Part model, mm, in its own coordinate system. A direction names the side the tool comes from. Round coordinates to 2 decimals unless told otherwise and drop trailing zeros. Write each loop counter-clockwise with the first axis right and the second up, starting at its lowest first coordinate (ties: lowest second). Pieces come first, ordered by that corner, then holes.
```python
from build123d import *

# Parameters (mm, degrees)
F0_R     = 6
F1_DEPTH = 10


with BuildPart() as f1:
    # F0 (on Front) → F1 (new body)
    with BuildSketch(Plane.XZ):
        with BuildLine():
            Line((0, 15), (0, 0))
            Line((0, 0), (55, 0))
            Line((55, 0), (80, 0))
            Line((80, 0), (80, 40))
            Line((80, 40), (70, 40))
            Line((70, 40), (70, 74.051529))
            ThreePointArc((70, 74.051529), (66.311166, 78.381983), (60.857511, 80))
            Line((60.857511, 80), (10, 80))
            Line((10, 80), (10, 15))
            Line((10, 15), (0, 15))
        make_face()
        with Locations((30, 15.13609)):
            Circle(F0_R, mode=Mode.SUBTRACT)
        with Locations((55, 15)):
            Circle(F0_R, mode=Mode.SUBTRACT)
        with Locations((30, 40)):
            Circle(F0_R, mode=Mode.SUBTRACT)
        with Locations((30, 65.102487)):
            Circle(F0_R, mode=Mode.SUBTRACT)
        with Locations((55, 40)):
            Circle(F0_R, mode=Mode.SUBTRACT)
        with Locations((55, 65.307461)):
            Circle(F0_R, mode=Mode.SUBTRACT)
    extrude(amount=F1_DEPTH)


solid = f1.part
```
Q1. Drop a flat-ended pin along its axis: pin 1 (5 mm diameter, centred on x = 6.5, y = -5.5, fed in from +Z). Give the stop position or say it passes through.
Values follow:
pin 1: stops at z = 15
Q2. Cut at B-B on z = 11. Write the cut outline in (x, y).
Values follow:
outline: (0, -10) - (25.65, -10) - (25.65, 0) - (0, 0) - close; (34.35, -10) - (50.53, -10) - (50.53, 0) - (34.35, 0) - close; (59.47, -10) - (80, -10) - (80, 0) - (59.47, 0) - close
Q3. Wall check: L1, parallel to Z at x = 55, y = -4.25; L2, parallel to Z at x = 30, y = -5.25; L3, parallel to X at y = -1, z = 41. Give the ranges that are in metal, low to high.
Values follow:
L1: z = 0 to 9, 21 to 34, 46 to 59.31, 71.31 to 80
L2: z = 0 to 9.14, 21.14 to 34, 46 to 59.1, 71.1 to 80
L3: x = 10 to 24.08, 35.92 to 49.08, 60.92 to 70
Q4. Cut at A-A on x = 55. Write the cut outline in (y, z), plus the area to 3 significant figures.
Values follow:
outline: (-10, 0) - (0, 0) - (0, 9) - (-10, 9) - close; (-10, 21) - (0, 21) - (0, 34) - (-10, 34) - close; (-10, 46) - (0, 46) - (0, 59.31) - (-10, 59.31) - close; (-10, 71.31) - (0, 71.31) - (0, 80) - (-10, 80) - close
area: 440 mm2
Q5. Cut at D-D on z = 36.5. Write the cut outline in (x, y), plus the area to 3 significant figures.
Values follow:
outline: (10, -10) - (25.13, -10) - (25.13, 0) - (10, 0) - close; (34.87, -10) - (50.13, -10) - (50.13, 0) - (34.87, 0) - close; (59.87, -10) - (80, -10) - (80, 0) - (59.87, 0) - close
area: 505 mm2
Q6. Cut at C-C on y = -7.25. Write the cut outline in (x, z), plus the area to 3 significant figures.
Values follow:
outline: (0, 0) - (80, 0) - (80, 40) - (70, 40) - (70, 74.05) arc R10 ccw to (60.86, 80) - (10, 80) - (10, 15) - (0, 15) - close; hole circle Ø12 at (30, 15.14); hole circle Ø12 at (30, 40); hole circle Ø12 at (30, 65.1); hole circle Ø12 at (55, 15); hole circle Ø12 at (55, 40); hole circle Ø12 at (55, 65.31)
area: 4,660 mm2
Q7. Mould opens along X. For faces 1 (the cylindrical face through (50.578, -4.93, 69.363)), 2 (the flat face through (10, -5, 48)), 3 (the flat face through (5, -5, 15)) say: +X half, -X half, draft (parallel to the pull), parting line (faces both ways), or undercut.
Values follow:
face 1: undercut
face 2: -X half
face 3: draft
Q8. Which spindle directions (+Z, -Z, +X, -X, +Y, -Y) get a long thin tool onto all of the face, cutting with end or side? Do faces 4 (the cylindrical face through (49, -5, 15)), 5 (the flat face through (70, -5, 57)). Say none if no direction does.
Values follow:
face 4: +Y, -Y
face 5: +Z, +X, +Y, -Y
